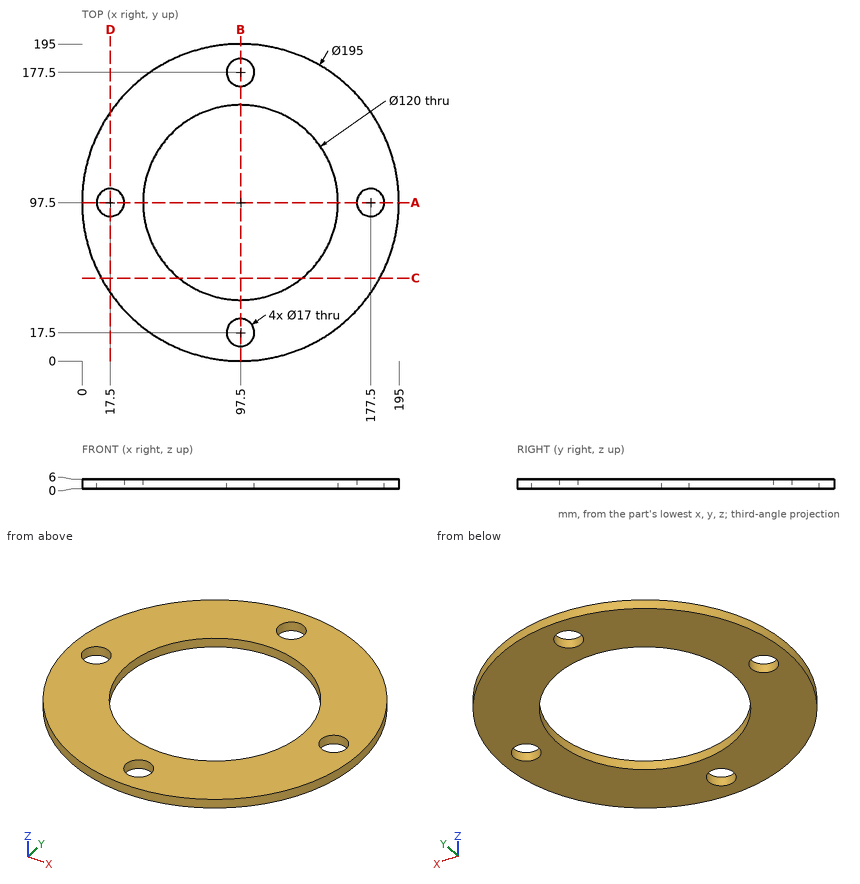
Geometry check sheet. Reference: drawing and pictorial views, mm from the part's lowest x, y, z. Give positions to 0.01 mm unless a question says otherwise; leave off trailing zeros. Order: outer loops, then holes, each group sorted by start corner. A loop starts at its lowest first (then second) coordinate and runs counter-clockwise, first axis right, second up. Notation, with made-up numbers: M 57,43 L 114,43 A8 ccw 114,48 Z; hole C 76,-39.5 d3. An arc over 180 degrees is marked long. Return JSON: item names as keys, results as strings. Group by question number.
1) Scan lines: line 1 (X direction, y = 97, z = 1.5); line 2 (X direction, y = 91, z = 4.3); line 3 (Y direction, x = 100, z = 4.8). Record each from-to range of solid material in increasing order.
2) Go/stop test with flat-tipped pins: pin 1 Ø1 at (y, z) = (172.5, 0.5) entering from +X; pin 2 Ø13.5 at (x, y) = (97.5, 17.5) entering from +Z. Record where each tip stops, or that it passes through.
3) Section check A-A on y = 97.5. Record the cut outline in (x, z), and give its area (3 significant figures).
4) Section check C-C on y = 51. Record the cut outline in (x, z).
5) Section check D-D on x = 17.5. Record the cut outline in (y, z).
Answer block:
{
 "1": {"line 1": "x = 0 to 9.01, 25.99 to 37.5, 157.5 to 169.01, 185.99 to 195", "line 2": "x = 0.22 to 12.02, 22.98 to 37.85, 157.15 to 172.02, 182.98 to 194.78", "line 3": "y = 0.03 to 9.38, 25.62 to 37.55, 157.45 to 169.38, 185.62 to 194.97"},
 "2": {"pin 1": "stops at x = 160.4", "pin 2": "passes through"},
 "3": {"outline": "M 0,0 L 9,0 L 9,6 L 0,6 Z; M 26,0 L 37.5,0 L 37.5,6 L 26,6 Z; M 157.5,0 L 169,0 L 169,6 L 157.5,6 Z; M 186,0 L 195,0 L 195,6 L 186,6 Z", "area": "246 mm^2"},
 "4": {"outline": "M 11.8,0 L 59.58,0 L 59.58,6 L 11.8,6 Z; M 135.42,0 L 183.2,0 L 183.2,6 L 135.42,6 Z"},
 "5": {"outline": "M 41.77,0 L 89,0 L 89,6 L 41.77,6 Z; M 106,0 L 153.23,0 L 153.23,6 L 106,6 Z"}
}
